```python
from build123d import *

# Parameters (mm, degrees)
PAD_DEPTH              = 1
PAD001_DEPTH           = 6.8
PAD001_DEPTH_BACK      = 6.8
CYLINDER_R             = 0.4
CYLINDER_DEPTH         = 13.6
CYLINDER001_R          = 1
CYLINDER001_DEPTH      = 0.5
LINEARPATTERN_COUNT    = 9
LINEARPATTERN_PITCH    = 3.75
CYLINDER002_R          = 0.7
CYLINDER002_DEPTH      = 0.5
LINEARPATTERN001_COUNT = 9
LINEARPATTERN001_PITCH = 3.75
CHAMFER_SIZE           = 0.4


with BuildPart() as part:
    # Sketch → Pad (new body)
    with BuildSketch(Plane.XY):
        with BuildLine():
            Line((0, 10), (80, 10))
            Line((80, 10), (80, -10))
            Line((0, -10), (80, -10))
            ThreePointArc((0, 10), (-10, 0), (0, -10))
        make_face()
    extrude(amount=PAD_DEPTH)

    # Sketch002 (on Sketch) → Pad001 (join, two sides)
    with BuildSketch(Plane.XZ) as pad001_sk:
        with BuildLine():
            Line((80, 0), (82.25, 0))
            ThreePointArc((82.25, 0), (83.090481, 2.14888), (80.972274, 1.233843))
            ThreePointArc((80, 1), (80.503859, 1.043236), (80.972274, 1.233843))
            Line((80, 1), (80, 0))
        make_face()
    extrude(amount=PAD001_DEPTH)
    extrude(pad001_sk.sketch, amount=-PAD001_DEPTH_BACK)

    # Cylinder → Cylinder (cut)
    with BuildSketch(Plane(origin=(82.25, 6.8, 1.25), x_dir=(1, 0, 0), z_dir=(0, -1, 0))):
        Circle(CYLINDER_R)
    extrude(amount=CYLINDER_DEPTH, mode=Mode.SUBTRACT)

    # Cylinder001 → Cylinder001 (cut)
    with BuildSketch(Plane.XY.offset(0.5)):
        Circle(CYLINDER001_R)
    cylinder001 = extrude(amount=CYLINDER001_DEPTH, mode=Mode.SUBTRACT)

    # LinearPattern: Cylinder001 ×9
    with Locations(*[(i * LINEARPATTERN_PITCH, 0, 0) for i in range(1, LINEARPATTERN_COUNT)]):
        add(cylinder001, mode=Mode.SUBTRACT)

    # Cylinder002 → Cylinder002 (cut)
    with BuildSketch(Plane.XY):
        Circle(CYLINDER002_R)
    cylinder002 = extrude(amount=CYLINDER002_DEPTH, mode=Mode.SUBTRACT)

    # LinearPattern001: Cylinder002 ×9
    with Locations(*[(i * LINEARPATTERN001_PITCH, 0, 0) for i in range(1, LINEARPATTERN001_COUNT)]):
        add(cylinder002, mode=Mode.SUBTRACT)

    # Chamfer
    chamfer_edges = [part.edges().sort_by_distance(p)[0] for p in [
        (40, -10, 1),
        (40, 10, 1),
        (-10, 0, 1),
        (40, 10, 0),
        (40, -10, 0),
        (-10, 0, 0),
    ]]
    chamfer(chamfer_edges, length=CHAMFER_SIZE)


solid = part.part
```
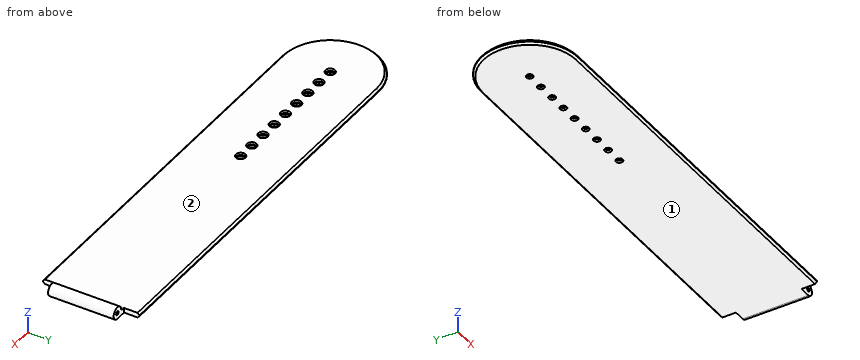
The model under review builds one solid part; all positions refer to its coordinate system, in mm. Face numbers are marked on the shaded views. A direction names the side the tool comes from. Round coordinates to 2 decimals unless told otherwise and drop trailing zeros. Loops run counter-clockwise (first coordinate to the right, second up) from the corner with the lowest first, then second, coordinate; pieces in that order, holes last.
Item 1: Clearance check with flat-ended pins moving along their axes: pin 1 Ø12 at (x, y) = (67.5, 4.5) entering from +Z; pin 2 Ø0.7 at (x, z) = (81.5, 1) entering from -Y; pin 3 Ø0.6 at (x, y) = (26.5, -0.5) entering from +Z; pin 4 Ø1.1 at (x, y) = (22.5, 0) entering from -Z (1 decimal). State where each tip first meets the part, or that it passes through.
Determined:
pin 1: stops at z = 1
pin 2: stops at y = -6.8
pin 3: stops at z = 0.5
pin 4: passes through
Item 2: For line 1 (Z direction, x = 26, y = 5.25); line 2 (Y direction, x = 26.25, z = 0.7); line 3 (Y direction, x = 11, z = 0.95), list the stretches that pass through material, from the lowest coordinate up.
Determined:
line 1: z = 0 to 1
line 2: y = -9.9 to -1, 1 to 9.9
line 3: y = -9.65 to -0.97, 0.97 to 9.65
Item 3: For the marked faces 1 and 2, list the 3-axis set-ups (+Z, -Z, +X, -X, +Y, -Y) from which the entire face can be reached by the end or side of a thin tool; tool diameter is ignored.
Determined:
face 1: -Z, +X, -X, +Y, -Y
face 2: +Z, -X, +Y, -Y
Item 4: Take a section at A-A (x = 62.5). Write out the cut boundary in (y, z), then the cut area to 3 significant figures.
Determined:
outline: (-10, 0.4) - (-9.6, 0) - (9.6, 0) - (10, 0.4) - (10, 0.6) - (9.6, 1) - (-9.6, 1) - (-10, 0.6) - close
area: 19.7 mm2
